For this review, take the finished solid that the model builds, in its own axes (mm). Face numbers are marked on the shaded views. A direction names the side the tool comes from. Round coordinates to 2 decimals unless told otherwise and drop trailing zeros. Order: outer loops, then holes, each group sorted by start corner. A loop starts at its lowest first (then second) coordinate and runs counter-clockwise, first axis right, second up. Notation, with made-up numbers: M 83.25,54 L 113.25,54 A29 cw 113.25,80 Z; hole C 59,-25 d5. An arc over 180 degrees is marked long. Use a Markdown table: item, result.
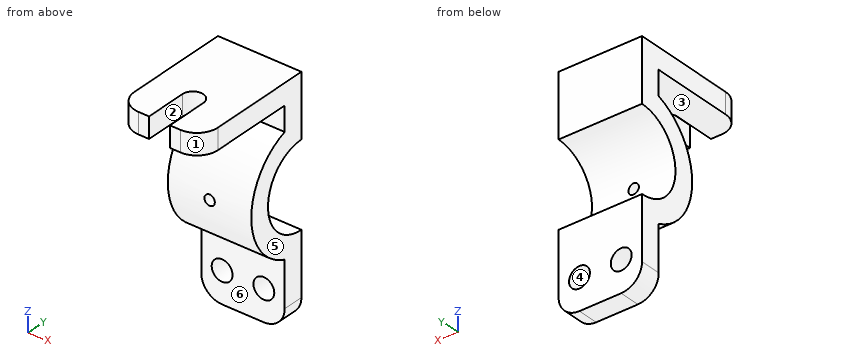
from build123d import *

# Parameters (mm, degrees)
BOSS_EXTRUDE1_DEPTH = 50.8
CUT_EXTRUDE1_DEPTH  = 22.86
CUT_EXTRUDE2_DEPTH  = 22.86
CUT_EXTRUDE3_DEPTH  = 22.86
SKETCH6_R           = 3.175
CUT_EXTRUDE4_DEPTH  = 60.96
CUT_EXTRUDE5_DEPTH  = 30.48
CUT_EXTRUDE6_DEPTH  = 30.48
SKETCH10_R          = 6.35
CUT_EXTRUDE7_DEPTH  = 30.48


with BuildPart() as part:
    # Sketch2 → Boss-Extrude1 (new body)
    with BuildSketch(Plane(origin=(0, 0, 0), x_dir=(0, 0, -1), z_dir=(1, 0, 0))):
        with BuildLine():
            Line((0, 0), (38.1, 0))
            ThreePointArc((38.1, 0), (63.5, -25.4), (88.9, 0))
            Line((88.9, 0), (139.7, 0))
            Line((139.7, 0), (139.7, -12.7))
            Line((139.7, -12.7), (99.421024484, -12.7))
            ThreePointArc((99.421024484, -12.7), (63.5, -38.1), (27.578975516, -12.7))
            Line((27.578975516, -12.7), (12.7, -12.7))
            Line((12.7, -12.7), (12.7, -76.2))
            Line((12.7, -76.2), (0, -76.2))
            Line((0, -76.2), (0, 0))
        make_face()
    extrude(amount=BOSS_EXTRUDE1_DEPTH)

    # Sketch3 → Cut-Extrude1 (cut)
    with BuildSketch(Plane.XY):
        with BuildLine():
            Line((50.8, -63.5), (50.8, -76.2))
            Line((50.8, -76.2), (38.1, -76.2))
            ThreePointArc((38.1, -76.2), (47.080256121, -72.480256121), (50.8, -63.5))
        make_face()
    extrude(amount=-CUT_EXTRUDE1_DEPTH, mode=Mode.SUBTRACT)

    # Sketch4 → Cut-Extrude2 (cut)
    with BuildSketch(Plane.XY):
        with BuildLine():
            Line((0, -63.5), (0, -76.2))
            Line((0, -76.2), (12.7, -76.2))
            ThreePointArc((12.7, -76.2), (3.719743879, -72.480256121), (0, -63.5))
        make_face()
    extrude(amount=-CUT_EXTRUDE2_DEPTH, mode=Mode.SUBTRACT)

    # Sketch5 → Cut-Extrude3 (cut)
    with BuildSketch(Plane.XY):
        with BuildLine():
            Line((19.05, -76.2), (19.05, -50.8))
            ThreePointArc((19.05, -50.8), (25.4, -44.45), (31.75, -50.8))
            Line((31.75, -50.8), (31.75, -76.2))
            Line((31.75, -76.2), (19.05, -76.2))
        make_face()
    extrude(amount=-CUT_EXTRUDE3_DEPTH, mode=Mode.SUBTRACT)

    # Sketch6 → Cut-Extrude4 (cut)
    with BuildSketch(Plane(origin=(0, 0, 0), x_dir=(1, 0, 0), z_dir=(0, 1, 0))):
        with Locations((25.4, 63.5)):
            Circle(SKETCH6_R)
    extrude(amount=-CUT_EXTRUDE4_DEPTH, mode=Mode.SUBTRACT)

    # Sketch7 → Cut-Extrude5 (cut)
    with BuildSketch(Plane(origin=(0, 0, 0), x_dir=(1, 0, 0), z_dir=(0, 1, 0))):
        with BuildLine():
            Line((0, 127), (0, 139.7))
            Line((0, 139.7), (12.7, 139.7))
            ThreePointArc((12.7, 139.7), (3.719743879, 135.980256121), (0, 127))
        make_face()
    extrude(amount=-CUT_EXTRUDE5_DEPTH, mode=Mode.SUBTRACT)

    # Sketch9 → Cut-Extrude6 (cut)
    with BuildSketch(Plane(origin=(0, 0, 0), x_dir=(1, 0, 0), z_dir=(0, 1, 0))):
        with BuildLine():
            Line((50.8, 127), (50.8, 139.7))
            Line((50.8, 139.7), (38.1, 139.7))
            ThreePointArc((38.1, 139.7), (47.080256121, 135.980256121), (50.8, 127))
        make_face()
    extrude(amount=-CUT_EXTRUDE6_DEPTH, mode=Mode.SUBTRACT)

    # Sketch10 → Cut-Extrude7 (cut)
    with BuildSketch(Plane(origin=(0, 0, 0), x_dir=(1, 0, 0), z_dir=(0, 1, 0))):
        with Locations((38.1, 120.65)):
            Circle(SKETCH10_R)
        with Locations((12.7, 120.65)):
            Circle(SKETCH10_R)
    extrude(amount=-CUT_EXTRUDE7_DEPTH, mode=Mode.SUBTRACT)


solid = part.part
Q1. Machinability: for the marked faces 1, 2 and 3, which of the approach directions +Z, -Z, +X, -X, +Y, -Y give a long, thin tool a straight path to every point of the face, cutting with its end or side? Answer none if there is none.
Determined:
| item | result |
|---|---|
| face 1 | +Z, -Z, +X, -Y |
| face 2 | +Z, -Z, -Y |
| face 3 | +X, -X, -Y |
Q2. Add section D-D (y = -16). Write out the cut boundary in (x, z), then the cut area to 3 significant figures.
Determined:
| item | result |
|---|---|
| outline | M 0,-98.08 L 50.8,-98.08 L 50.8,-83.23 L 0,-83.23 Z; M 0,-43.77 L 50.8,-43.77 L 50.8,-28.92 L 0,-28.92 Z; M 0,-12.7 L 50.8,-12.7 L 50.8,0 L 0,0 Z |
| area | 2,150 mm^2 |
Q3. Clearance check with flat-ended pins moving along their axes: pin 1 (7.5 mm diameter, centred on x = 25.4, z = -63.5, fed in from +Y); pin 2 (2 mm diameter, centred on y = -16, z = -99.5, fed in from -X); pin 3 (15 mm diameter, centred on x = 25, y = -38.5, fed in from -Z); pin 4 (12 mm diameter, centred on x = 13.5, y = -29.5, fed in from -Z). State where each tip first meets the part, or that it passes through.
Determined:
| item | result |
|---|---|
| pin 1 | stops at y = -25.12 |
| pin 2 | passes through |
| pin 3 | stops at z = -85.65 |
| pin 4 | stops at z = -93.49 |
Q4. Add section B-B (z = -63.5). Write out the cut boundary in (x, y) (3 decimals), then the cut area to 3 significant figures.
Determined:
| item | result |
|---|---|
| outline | M 0,-38.1 L 22.225,-38.1 L 22.225,-25.4 L 0,-25.4 Z; M 28.575,-38.1 L 50.8,-38.1 L 50.8,-25.4 L 28.575,-25.4 Z |
| area | 565 mm^2 |
Q5. Add section C-C (x = 16.5). Write out the cut boundary in (y, z).
Determined:
| item | result |
|---|---|
| outline | M -76.2,-12.7 L -12.7,-12.7 L -12.7,-27.58 A38.1 ccw -12.7,-99.42 L -12.7,-115.56 L 0,-115.56 L 0,-88.9 A25.4 cw 0,-38.1 L 0,0 L -76.2,0 Z; M -12.7,-139.7 L 0,-139.7 L 0,-125.74 L -12.7,-125.74 Z |
Q6. Wall thickness on line 1 along X through (y, z) = (-7, -120.65); line 2 along Z through (x, y) = (38, -2); line 3 along Z through (x, y) = (21.5, -18): over which ranges is each line inside the solid? List them lowest first. Write a range as [from, to].
Determined:
| item | result |
|---|---|
| line 1 | x = [0, 6.35], [19.05, 31.75], [44.45, 50.8] |
| line 2 | z = [-139.7, -127], [-114.3, -88.82], [-38.18, 0] |
| line 3 | z = [-97.08, -81.42], [-45.58, -29.92], [-12.7, 0] |
Q7. Draft analysis for pull direction X (two halves, no side actions). For the marked faces 4, 5 and 6, state which applies: pulls with the +X half, pulls with the -X half, needs draft (parallel to the pull), parting line crosses it, or undercut.
Determined:
| item | result |
|---|---|
| face 4 | undercut |
| face 5 | pulls with the +X half |
| face 6 | needs draft |
Q8. Add section A-A (z = -120.65). Write out the cut boundary in (x, y), then the cut area to 3 significant figures.
Determined:
| item | result |
|---|---|
| outline | M 0,-12.7 L 6.35,-12.7 L 6.35,0 L 0,0 Z; M 19.05,-12.7 L 31.75,-12.7 L 31.75,0 L 19.05,0 Z; M 44.45,-12.7 L 50.8,-12.7 L 50.8,0 L 44.45,0 Z |
| area | 323 mm^2 |
